Verification items for the finished model (mm, model axes). A direction names the side the tool comes from. Round coordinates to 2 decimals unless told otherwise and drop trailing zeros. Order: outer loops, then holes, each group sorted by start corner. A loop starts at its lowest first (then second) coordinate and runs counter-clockwise, first axis right, second up. Notation, with made-up numbers: (55.5, -38.75) -> (81.5, -38.75) arc R14 cw to (81.5, -34.75) -> close; hole circle Ø9 at (65.25, -29). An arc over 180 degrees is marked (long way). Answer in a Markdown table with one row per item. Add a question column.
```python
from build123d import *

# Parameters (mm, degrees)
F1_DEPTH = 10


with BuildPart() as f1:
    # F0 (on Top) → F1 (new body)
    with BuildSketch(Plane.XY):
        with BuildLine():
            Line((0, 16.165808), (14, 8.082904))
            Line((14, 8.082904), (14, -8.082904))
            Line((14, -8.082904), (15.261739, -8.082904))
            ThreePointArc((15.261739, -8.082904), (15.916254, -8.422893), (16.014449, -9.153879))
            Line((16.014449, -9.153879), (14.985551, -12.011928))
            ThreePointArc((14.985551, -12.011928), (15.083746, -12.742914), (15.738261, -13.082904))
            Line((15.738261, -13.082904), (21.8, -13.082904))
            ThreePointArc((21.8, -13.082904), (22.365685, -12.848589), (22.6, -12.282904))
            Line((22.6, -12.282904), (22.6, -8.882904))
            ThreePointArc((22.6, -8.882904), (22.834315, -8.317218), (23.4, -8.082904))
            Line((23.4, -8.082904), (25, -8.082904))
            Line((25, -8.082904), (25, -7.882904))
            Line((25, -7.882904), (25, 0))
            ThreePointArc((25, 0), (0, 25), (-25, 0))
            Line((-25, 0), (-25, -7.882904))
            Line((-25, -7.882904), (-25, -8.082904))
            Line((-25, -8.082904), (-23.4, -8.082904))
            ThreePointArc((-23.4, -8.082904), (-22.834315, -8.317218), (-22.6, -8.882904))
            Line((-22.6, -8.882904), (-22.6, -12.282904))
            ThreePointArc((-22.6, -12.282904), (-22.365685, -12.848589), (-21.8, -13.082904))
            Line((-21.8, -13.082904), (-15.738261, -13.082904))
            ThreePointArc((-15.738261, -13.082904), (-15.083746, -12.742914), (-14.985551, -12.011928))
            Line((-14.985551, -12.011928), (-16.014449, -9.153879))
            ThreePointArc((-16.014449, -9.153879), (-15.916254, -8.422893), (-15.261739, -8.082904))
            Line((-15.261739, -8.082904), (-14, -8.082904))
            Line((-14, -8.082904), (-14, 8.082904))
            Line((-14, 8.082904), (0, 16.165808))
        make_face()
    extrude(amount=F1_DEPTH)


solid = f1.part
```
1) Draft check along Y on faces 1 (the face through (5, 15, 0)), 2 (the face through (-19, -13.083, 5)), 3 (the face through (-15.493, -10.603, 4.93)), 4 (the face through (15, -8.083, 5)). Enter one of: +Y half, -Y half, draft (parallel to the pull), parting line (faces both ways), or undercut.
2) Thickness scan on L1, parallel to X at y = -1, z = 6; L2, parallel to X at y = 5.5, z = 8.5; L3, parallel to Y at x = 23, z = 5.25. Record the ranges inside material, lowest first. Write a range as [from, to].
3) Cross-section at C-C, the plane x = -20. Record the boundary of the cut face in (y, z), and give its area (3 significant figures).
4) Cross-section at B-B, the plane z = 7.5. Record the boundary of the cut face in (x, y), and give its area (3 significant figures).
5) Tool access check on faces 5 (the face through (24, -8.083, 5)), 6 (the face through (-15, -8.083, 5)), 7 (the face through (-24, -8.083, 5)), 8 (the face through (-7.098, 12.068, 4.93)), 9 (the face through (-25, -4, 5)). Record the directions out of +Z, -Z, +X, -X, +Y, -Y that give a thin tool (end or side, any length) a straight path to the whole face; none if there is none.
6) Depth check by flat-ended pin: P1, Ø4, axis at x = 19.5, y = 16.5, coming from the -Z side; P2, Ø1.8, axis at x = -24, z = 5, coming from the -Y side; P3, Ø3.5, axis at y = -10.5, z = 5, coming from the -X side; P4, Ø2, axis at y = 3, z = 2.5, coming from the -X side. Enter the tip coordinate at first touch or a pass-through.
7) Cross-section at A-A, the plane y = -3.5. Record the boundary of the cut face in (x, z), and give its area (3 significant figures).
8) Cross-section at D-D, the plane y = 5.5. Record the boundary of the cut face in (x, z).
Results below:
| question | item | result |
|---|---|---|
| 1 | face 1 | draft |
| 1 | face 2 | -Y half |
| 1 | face 3 | undercut |
| 1 | face 4 | undercut |
| 2 | L1 | [-25, -14], [14, 25] |
| 2 | L2 | [-24.39, -14], [14, 24.39] |
| 2 | L3 | [-8.19, 9.8] |
| 3 | outline | (-13.08, 0) -> (15, 0) -> (15, 10) -> (-13.08, 10) -> close |
| 3 | area | 281 mm² |
| 4 | outline | (-25, -8.08) -> (-23.4, -8.08) arc R0.8 cw to (-22.6, -8.88) -> (-22.6, -12.28) arc R0.8 ccw to (-21.8, -13.08) -> (-15.74, -13.08) arc R0.8 ccw to (-14.99, -12.01) -> (-16.01, -9.15) arc R0.8 cw to (-15.26, -8.08) -> (-14, -8.08) -> (-14, 8.08) -> (0, 16.17) -> (14, 8.08) -> (14, -8.08) -> (15.26, -8.08) arc R0.8 cw to (16.01, -9.15) -> (14.99, -12.01) arc R0.8 ccw to (15.74, -13.08) -> (21.8, -13.08) arc R0.8 ccw to (22.6, -12.28) -> (22.6, -8.88) arc R0.8 cw to (23.4, -8.08) -> (25, -8.08) -> (25, 0) arc R25 ccw to (-25, 0) -> close |
| 4 | area | 891 mm² |
| 5 | face 5 | +Z, -Z, +X, -Y |
| 5 | face 6 | +Z, -Z |
| 5 | face 7 | +Z, -Z, -X, -Y |
| 5 | face 8 | +Z, -Z, -Y |
| 5 | face 9 | +Z, -Z, -X, +Y, -Y |
| 6 | P1 | z = 0 |
| 6 | P2 | y = -8.14 |
| 6 | P3 | x = -22.61 |
| 6 | P4 | x = -24.92 |
| 7 | outline | (-25, 0) -> (-14, 0) -> (-14, 10) -> (-25, 10) -> close; (14, 0) -> (25, 0) -> (25, 10) -> (14, 10) -> close |
| 7 | area | 220 mm² |
| 8 | outline | (-24.39, 0) -> (-14, 0) -> (-14, 10) -> (-24.39, 10) -> close; (14, 0) -> (24.39, 0) -> (24.39, 10) -> (14, 10) -> close |
